Check sheet for the modelled part. Datum: model origin and axes. Units: mm. Face numbers are marked on the shaded views. A direction names the side the tool comes from. Give positions to 0.01 mm unless a question says otherwise; leave off trailing zeros. Order: outer loops, then holes, each group sorted by start corner. A loop starts at its lowest first (then second) coordinate and runs counter-clockwise, first axis right, second up.
```python
from build123d import *

# Parameters (mm, degrees)
ESQUISSE2_W             = 6.5
ESQUISSE2_H             = 7.5
ENL_V_MAT_EXTRU_1_DEPTH = 20


with BuildPart() as part:
    # Esquisse1 → R_volution1 (revolve)
    with BuildSketch(Plane.XY, mode=Mode.PRIVATE) as r_volution1_sk:
        with BuildLine():
            Line((-17, 5.5), (-17, 3.85))
            Line((-17, 3.85), (0, 3.85))
            Line((0, 3.85), (0, 5.5))
            Line((0, 5.5), (-0.5, 6))
            Line((-0.5, 6), (-11.68337521, 6))
            ThreePointArc((-11.68337521, 6), (-13.341687605, 5.5), (-15, 6))
            Line((-15, 6), (-16.5, 6))
            Line((-16.5, 6), (-17, 5.5))
        make_face()
    revolve(r_volution1_sk.sketch.rotate(Axis((-34.750549451, 0, 0), (1, 0, 0)), 90), axis=Axis((-34.750549451, 0, 0), (1, 0, 0)))

    # Esquisse2 → Enl_v. mat.-Extru.1 (cut, through all)
    with BuildSketch(Plane(origin=(0, 0, 0), x_dir=(0, 0, -1), z_dir=(1, 0, 0))):
        Rectangle(ESQUISSE2_W, ESQUISSE2_H)
    extrude(amount=-ENL_V_MAT_EXTRU_1_DEPTH, mode=Mode.SUBTRACT)


solid = part.part
```
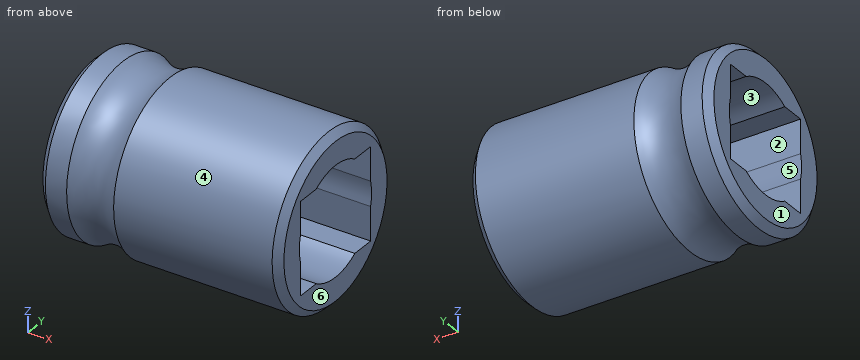
(1) Release check for a two-part mould opening along Y. For the marked faces 1, 2, 3 and 4 record: released by +Y, released by -Y, zero draft, split by the parting line, or undercut.
Response values:
face 1: zero draft
face 2: undercut
face 3: undercut
face 4: split by the parting line
(2) Cross-section at B-B on y = 0. Enter the section's corners in (x, z).
Response values:
outline: (-17, -5.5) - (-16.5, -6) - (-15, -6) arc R3 cw to (-11.68, -6) - (-0.5, -6) - (0, -5.5) - (0, -3.85) - (-17, -3.85) - close; (-17, 3.85) - (0, 3.85) - (0, 5.5) - (-0.5, 6) - (-11.68, 6) arc R3 cw to (-15, 6) - (-16.5, 6) - (-17, 5.5) - close
(3) Set-up check for the marked faces 5 and 6: record each of +Z, -Z, +X, -X, +Y, -Y from which the full face is reachable in a straight line by a thin tool's end or side.
Response values:
face 5: +X, -X
face 6: +Z, -Z, +X, +Y, -Y
(4) Cross-section at D-D on x = -14.75. Enter the section's corners in (y, z), then the cut area to 3 significant figures.
Response values:
outline: circle Ø11.7 at (0, 0); hole (-3.75, -3.25) - (-2.06, -3.25) arc R3.85 ccw to (2.06, -3.25) - (3.75, -3.25) - (3.75, -0.87) arc R3.85 ccw to (3.75, 0.87) - (3.75, 3.25) - (2.06, 3.25) arc R3.85 ccw to (-2.06, 3.25) - (-3.75, 3.25) - (-3.75, 0.87) arc R3.85 ccw to (-3.75, -0.87) - close
area: 55.2 mm2
(5) Gauge pin test, flat ends, axial feed: pin 1 Ø6 at (x, z) = (-8.5, -4.5) entering from -Y; pin 2 Ø1.2 at (x, z) = (-8, -2) entering from +Y; pin 3 Ø1.9 at (x, y) = (-5, -3) entering from +Z. Record the tip position at first contact, or that the pin passes through.
Response values:
pin 1: stops at y = -5.81
pin 2: stops at y = 5.83
pin 3: stops at z = 5.64
(6) Material ranges on L1, parallel to Y at x = -1, z = -2.25; L2, parallel to Z at x = -1.5, y = 0.5; L3, parallel to Y at x = -7, z = 2.5, recorded low to high.
Response values:
L1: y = -5.56 to -3.75, 3.75 to 5.56
L2: z = -5.98 to -3.82, 3.82 to 5.98
L3: y = -5.45 to -3.75, 3.75 to 5.45
(7) Cross-section at A-A on x = -3. Enter the section's corners in (y, z).
Response values:
outline: circle Ø12 at (0, 0); hole (-3.75, -3.25) - (-2.06, -3.25) arc R3.85 ccw to (2.06, -3.25) - (3.75, -3.25) - (3.75, -0.87) arc R3.85 ccw to (3.75, 0.87) - (3.75, 3.25) - (2.06, 3.25) arc R3.85 ccw to (-2.06, 3.25) - (-3.75, 3.25) - (-3.75, 0.87) arc R3.85 ccw to (-3.75, -0.87) - close
